```python
from build123d import *

# Parameters (mm, degrees)
SKETCH1_W                 = 30
SKETCH1_H                 = 15
F_4_CLEARANCE_HOLE1_D     = 3.4
F_4_CLEARANCE_HOLE1_DEPTH = 15
HOLE1_D                   = 37
HOLE1_DEPTH               = 15
HOLE1_CBORE_D             = 46.98238
HOLE1_CBORE_DEPTH         = 11
CHAMFER1_SIZE             = 1.45


with BuildPart() as part:
    # Sketch1 → Revolve1 (revolve)
    with BuildSketch(Plane.XZ):
        with Locations((15, 7.5)):
            Rectangle(SKETCH1_W, SKETCH1_H)
    revolve(axis=Axis((0, 0, 15), (0, 0, -1)))

    # #4 Clearance Hole1
    with Locations(Plane(origin=(0, 0, 0), x_dir=(-1, 0, 0), z_dir=(0, 0, -1))):
        with Locations((-23.166179551, -13.375), (-23.166179551, 13.375), (0, 26.75), (23.166179551, -13.375), (0, -26.75), (23.166179551, 13.375)):
            Hole(F_4_CLEARANCE_HOLE1_D / 2, depth=F_4_CLEARANCE_HOLE1_DEPTH)

    # Hole1
    with Locations(Plane.XY.offset(15)):
        with Locations((0, 0)):
            CounterBoreHole(HOLE1_D / 2, HOLE1_CBORE_D / 2, HOLE1_CBORE_DEPTH, depth=HOLE1_DEPTH)

    # Chamfer1
    chamfer1_edges = [part.edges().sort_by_distance(p)[0] for p in [
        (-24.866179551, 13.375, 0),
        (-1.7, -26.75, 0),
        (-24.866179551, -13.375, 0),
        (-1.7, 26.75, 0),
        (21.466179551, 13.375, 0),
        (21.466179551, -13.375, 0),
    ]]
    chamfer(chamfer1_edges, length=CHAMFER1_SIZE)


solid = part.part
```
CAD build for the part. Positions are in the model's coordinates, mm. A direction names the side the tool comes from. Coordinates: 2 decimals unless noted, no trailing zeros. Order: outer loops, then holes, each group sorted by start corner. A loop starts at its lowest first (then second) coordinate and runs counter-clockwise, first axis right, second up.
(1) Saw through at A-A, the plane x = 0. Write the cut outline in (y, z).
Solution:
outline: (-30, 0) - (-29.9, 0) - (-28.45, 1.45) - (-28.45, 15) - (-30, 15) - close; (-25.05, 1.45) - (-23.6, 0) - (-18.5, 0) - (-18.5, 4) - (-23.49, 4) - (-23.49, 15) - (-25.05, 15) - close; (18.5, 0) - (23.6, 0) - (25.05, 1.45) - (25.05, 15) - (23.49, 15) - (23.49, 4) - (18.5, 4) - close; (28.45, 1.45) - (29.9, 0) - (30, 0) - (30, 15) - (28.45, 15) - close
(2) Which spindle directions (+Z, -Z, +X, -X, +Y, -Y) get a long thin tool onto all of the face, cutting with end or side? Do faces 5 (the face through (21.468, 13.45, 8.32)), 6 (the face through (10.84, -20.84, 9.58)). Say none if no direction does.
Solution:
face 5: +Z, -Z
face 6: +Z
(3) Saw through at C-C, the plane z = 10.5. Write the cut outline in (x, y) (3 decimals), and give its area (3 significant figures).
Solution:
outline: circle Ø60 at (0, 0); hole circle Ø3.4 at (-23.166, -13.375); hole circle Ø3.4 at (-23.166, 13.375); hole circle Ø46.982 at (0, 0); hole circle Ø3.4 at (0, -26.75); hole circle Ø3.4 at (0, 26.75); hole circle Ø3.4 at (23.166, -13.375); hole circle Ø3.4 at (23.166, 13.375)
area: 1,040 mm2
(4) Mould opens along Y. For faces 1 (the face through (-0.221, -25.064, 8.32)), 2 (the face through (-29.97, -1.32, 7.6)), 3 (the face through (-21.596, 12.724, 8.32)), 4 (the face through (14, 13, 0)) say: released by +Y, released by -Y, zero draft, split by the parting line, or undercut.
Solution:
face 1: undercut
face 2: split by the parting line
face 3: undercut
face 4: zero draft
(5) Saw through at D-D, the plane x = -6. Write the cut outline in (y, z), and give its area (3 significant figures).
Solution:
outline: (-29.39, 0) - (-17.5, 0) - (-17.5, 4) - (-22.71, 4) - (-22.71, 15) - (-29.39, 15) - close; (17.5, 0) - (29.39, 0) - (29.39, 15) - (22.71, 15) - (22.71, 4) - (17.5, 4) - close
area: 242 mm2
(6) Drill centre lines: L1, parallel to Y at x = 0, z = 13.25; L2, parallel to Y at x = -22.5, z = 3; L3, parallel to Y at x = 24, z = 11. Where is each one in solid material? Low to high.
Solution:
L1: y = -30 to -28.45, -25.05 to -23.49, 23.49 to 25.05, 28.45 to 30
L2: y = -19.84 to -14.94, -11.81 to 11.81, 14.94 to 19.84
L3: y = -18 to -14.86, -11.89 to 11.89, 14.86 to 18
(7) Saw through at B-B, the plane y = 0. Write the cut outline in (x, z), and give its area (3 significant figures).
Solution:
outline: (-30, 0) - (-18.5, 0) - (-18.5, 4) - (-23.49, 4) - (-23.49, 15) - (-30, 15) - close; (18.5, 0) - (30, 0) - (30, 15) - (23.49, 15) - (23.49, 4) - (18.5, 4) - close
area: 235 mm2
(8) Pin check, flat tips, straight feed: pin 1 Ø8 at (x, z) = (-23, 11.5) entering from +Y; pin 2 Ø10 at (x, y) = (-7, 13) entering from +Z; pin 3 Ø2.5 at (x, y) = (-23.17, 13.38) entering from +Z; pin 4 Ø1 at (x, z) = (0.5, 12) entering from +Y. Stop position of each tip, or through.
Solution:
pin 1: stops at y = 23.22
pin 2: stops at z = 4
pin 3: passes through
pin 4: stops at y = 30
